The listing builds one solid part. Answer for the finished solid, in the listing's coordinates (mm). A direction names the side the tool comes from. Give positions to 0.01 mm unless a question says otherwise; leave off trailing zeros. Order: outer loops, then holes, each group sorted by start corner. A loop starts at its lowest first (then second) coordinate and runs counter-clockwise, first axis right, second up. Notation, with made-up numbers: (-37, 30) - (-30, 30) arc R21 ccw to (-30, 60) - close; hole circle Ø3 at (19.25, 58). An arc over 180 degrees is marked (long way). Answer in a Markdown table with one row per item. Add a question column.
```python
from build123d import *

# Parameters (mm, degrees)
SKETCH1_R           = 8.5
SKETCH1_R_2         = 7.35
BOSS_EXTRUDE3_DEPTH = 8.755
BOSS_EXTRUDE5_START = -0.3
SKETCH3_W           = 1.43994518
SKETCH3_H           = 4.3775
BOSS_EXTRUDE5_DEPTH = 1.1
CIRPATTERN1_COUNT   = 18
SKETCH6_R           = 8.5
CUT_EXTRUDE1_DEPTH  = 4.3775


with BuildPart() as part:
    # Sketch1 → Boss-Extrude3 (new body)
    with BuildSketch(Plane.XY):
        Circle(SKETCH1_R)
        Circle(SKETCH1_R_2, mode=Mode.SUBTRACT)
    extrude(amount=BOSS_EXTRUDE3_DEPTH)

    # Sketch3 → Boss-Extrude5 (add)
    with BuildSketch(Plane(origin=(0, 8.5, 0), x_dir=(1, 0, 0), z_dir=(0, 1, 0)).offset(BOSS_EXTRUDE5_START)):
        with Locations((0.71997259, -6.56625)):
            Rectangle(SKETCH3_W, SKETCH3_H)
    boss_extrude5 = extrude(amount=BOSS_EXTRUDE5_DEPTH)

    # CirPattern1: Boss-Extrude5 ×18 about axis
    cirpattern1_axis = Axis((0, 0, 0), (0, 0, 1))
    for i in range(1, CIRPATTERN1_COUNT):
        add(boss_extrude5.rotate(cirpattern1_axis, i * 360 / CIRPATTERN1_COUNT))

    # Sketch6 → Cut-Extrude1 (cut)
    with BuildSketch(Plane(origin=(0, 0, 0), x_dir=(-1, 0, 0), z_dir=(0, 0, -1))):
        Circle(SKETCH6_R)
    extrude(amount=-CUT_EXTRUDE1_DEPTH, mode=Mode.SUBTRACT)


solid = part.part
```
(1) Straight lines are drawn through the part: line 1 (X direction, y = 0, z = 7); line 2 (X direction, y = 6, z = 6.3); line 3 (Y direction, x = -2.25, z = 6.9). For each, find the intervals that lie inside material, in ascending order.
(2) For faces 5 (the face through (-8.47, 0.73, 6.54)), 6 (the face through (-6.02, 6, 6.54)), 7 (the face through (-2.193, -8.212, 6.536)), determine the directions among +Z, -Z, +X, -X, +Y, -Y from which every point of the face is accessible in a straight line to the end or side of a thin tool.
(3) Each of these flat-tipped pins is pushed along its axis until it touches: P1, Ø1.5, axis at x = 5, y = -1, coming from the +Z side; P2, Ø1, axis at x = -7, z = 6, coming from the -Y side; P3, Ø0.6, axis at y = 9, z = 6, coming from the -X side; P4, Ø2, axis at x = 6.5, z = 8, coming from the -Y side. Where does it stop, or does it pass through?
(4) Find section A-A, the plane y = 7.75. Write down the section's boundary in (x, z) (1 decimal).
(5) Find section B-B, the plane x = -0.25. Write down the section's boundary in (y, z) (1 decimal), plus the area to 3 significant figures.
(6) The mould has two halves that part along X. Classify faces 1 (the face through (6.52, 6.67, 6.54)), 2 (the face through (6.02, -6, 6.54)), 3 (the face through (-1, -9.3, 7)), 4 (the face through (-7.7, 5.26, 6.54)): +X half, -X half, draft (parallel to the pull), parting line (faces both ways), or undercut.
Answer key:
| question | item | result |
|---|---|---|
| 1 | line 1 | -8.5 to -7.35, 7.35 to 8.5 |
| 1 | line 2 | -6.02 to -4.25, 4.25 to 6.91 |
| 1 | line 3 | -8.2 to -7, 7 to 9.08 |
| 2 | face 5 | +Z, -Z, -X |
| 2 | face 6 | +Z, -Z |
| 2 | face 7 | +Z, -Z, -Y |
| 3 | P1 | through |
| 3 | P2 | y = -6.69 |
| 3 | P3 | x = -3.18 |
| 3 | P4 | y = -7.53 |
| 4 | outline | (-5.2, 4.4) - (-4.6, 4.4) - (-4.6, 8.8) - (-5.2, 8.8) - close; (-3.5, 4.4) - (4.4, 4.4) - (4.4, 8.8) - (-3.5, 8.8) - close |
| 5 | outline | (-9.3, 4.4) - (-7.3, 4.4) - (-7.3, 8.8) - (-9.3, 8.8) - close; (7.3, 4.4) - (8.5, 4.4) - (8.5, 8.8) - (7.3, 8.8) - close |
| 5 | area | 13.6 mm² |
| 6 | face 1 | +X half |
| 6 | face 2 | undercut |
| 6 | face 3 | draft |
| 6 | face 4 | -X half |
